Autodesk Inventor part; units mm, degrees
ref_plane "作業平面1" through (-60, -5.7151, 26) normal (0, 0, -1) x (0, 1, 0)
ref_plane "YZ Plane" through (0, 0, 0) normal (1, 0, 0) x (0, 1, 0)
ref_plane "XZ Plane" through (0, 0, 0) normal (0, 1, 0) x (-1, 0, 0)
sketch "スケッチ1" plane through (0, 0, 0) normal (0, 0, 1) x (1, 0, 0)
  circle A0 centre (-4.6538, 21.3462) radius 1.1
  circle A1 centre (-19.6538, 21.3462) radius 1.1
  line L0 (0.5, 16.7574) -> (0.5, 6.421)
  arc A2 (-3.1924, 5.3553) -> (0.5, 6.421) centre (-1.5, 6.421) ccw
  arc A3 (-3.1924, 5.3553) -> (-13.8372, 15.4455) centre (-28.2569, -10.4267) ccw
  arc A4 (-12.8636, 19.1925) -> (-13.8372, 15.4455) centre (-12.8636, 17.1925) ccw
  line L1 (-12.8636, 19.1925) -> (-2.3985, 19.1925)
  arc A5 (-1.3325, 18.8847) -> (-2.3985, 19.1925) centre (-2.3985, 17.1925) ccw
  arc A6 (-1.3325, 18.8847) -> (-0.8333, 18.643) centre (0, 21) ccw
  arc A7 (0.5, 16.7574) -> (-0.8333, 18.643) centre (-1.5, 16.7574) ccw
  arc A8 (-2.3454, -0.8655) -> (2.5, 0) centre (0, 0) ccw
  line L2 (2.5, 0) -> (2.5, 16.5)
  arc A9 (4.5, 18.5) -> (2.5, 16.5) centre (4.5, 16.5) ccw
  line L3 (4.5, 18.5) -> (21, 18.5)
  arc A10 (21, 18.5) -> (21, 23.5) centre (21, 21) ccw
  line L4 (21, 23.5) -> (-25, 23.5)
  arc A11 (-25, 23.5) -> (-59.8955, -2.5) centre (-25, -12.9173) ccw
  arc A12 (-59.8955, -2.5) -> (-55.0727, -3.8137) centre (-57.5, -3.2151) ccw
  arc A13 (-2.3454, -0.8655) -> (-55.0727, -3.8137) centre (-28.2569, -10.4267) ccw
  circle A14 centre (0, 0) radius 1.1
  circle A15 centre (-47.2894, 12.7841) radius 1.1
  circle A16 centre (-29.7988, 20.1536) radius 1.1
  circle A17 centre (0, 21) radius 1.1
  circle A18 centre (-57.5, -3.2151) radius 1.1
  circle A19 centre (21, 21) radius 1.1
  line L5 (-12.8636, 19.1925) -> (-20.8636, 19.1925)
  line L6 (-33.6212, 16.6665) -> (-20.8636, 19.1925)
  circle A20 centre (-57.5, -3.2151) radius 0.8
  circle A21 centre (-47.2894, 12.7841) radius 0.8
  circle A22 centre (-29.7988, 20.1536) radius 0.8
  circle A23 centre (-19.6538, 21.3462) radius 0.8
  circle A24 centre (-4.6538, 21.3462) radius 0.8
  circle A25 centre (-4.6538, 21.3462) radius 2.1538
  point P0 (0, 0)
  point P1 (-4.6538, 19.1925)
  point P2 (-4.6538, 23.5)
  dimension "d0" = 8
  dimension "d1" = 1.6
  dimension "d2" = 1.6
  dimension "d3" = 1.6
  dimension "d4" = 1.6
  dimension "d5" = 1.6
ref_plane "作業平面1" through (-60, -5.7151, 26) normal (0, 0, -1) x (0, 1, 0)
extrude "押し出し1" add sketch "スケッチ1" along normal up to surface (26 mm away) contours A0 | A1 | L5 L6 A13 A12 A11 L4 A25 L1 | A25 | A15 | A16 | A18
fillet "フィレット1" radius 2 1 edges at (-20.8636, 19.1925, 13)
properties part number "tesaki_sukima" material "ABS プラスチック"
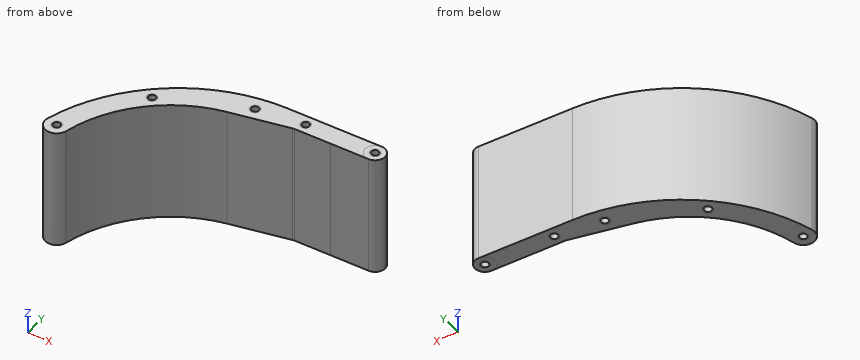
Design review of the part built by this model. Coordinates are the model's own, in mm. Coordinates: 2 decimals unless noted, no trailing zeros. Loops run counter-clockwise (first coordinate to the right, second up) from the corner with the lowest first, then second, coordinate; pieces in that order, holes last. Notation, with made-up numbers: M 56,9.25 L 94,9.25 A30 ccw 94,47.25 Z; hole C -13,-14.5 d2. An arc over 180 degrees is marked long. Answer as CSV lines item,"result".
Item 1: For probe 1 along Y at (x, z) = (-20.5, 6.25); probe 2 along X at (y, z) = (-3.5, 19); probe 3 along Y at (x, z) = (-57.5, 14.5), list the stretches that pass through material, from the lowest coordinate up.
Answer list:
probe 1,"19.19 to 23.5"
probe 2,"-59.98 to -58.25, -56.75 to -54.99"
probe 3,"-5.72 to -4.02, -2.42 to 3.51"
Item 2: Add section D-D on x = -42. State the section outline as (y, z) points.
Answer list:
outline,"M 13.53,0 L 19.29,0 L 19.29,26 L 13.53,26 Z"
Item 3: Add section B-B on z = 8.5. State the section outline as (x, y) points, plus the area to 3 significant figures.
Answer list:
outline,"M -59.9,-2.5 A2.5 ccw long -55.07,-3.81 A27.62 cw -33.62,16.67 L -21.06,19.15 A2 cw -20.67,19.19 L -4.65,19.19 A2.15 ccw -4.65,23.5 L -25,23.5 A36.42 ccw Z; hole C -57.5,-3.22 d1.6; hole C -47.29,12.78 d1.6; hole C -29.8,20.15 d1.6; hole C -19.65,21.35 d1.6; hole C -4.65,21.35 d1.6"
area,"316 mm²"
Item 4: Add section C-C on y = 0.25. State the section outline as (x, z) points, plus the area to 3 significant figures.
Answer list:
outline,"M -58.95,0 L -53.73,0 L -53.73,26 L -58.95,26 Z"
area,"136 mm²"
Item 5: For P1, Ø10, axis at x = -37, z = 22, coming from the -Y side; P2, Ø3, axis at y = 6, z = 20.5, coming from the +X side; P3, Ø2.5, axis at x = -17, z = 15, coming from the -Y side, all flat-tipped, find the tip position at first contact; note any pin that passes through.
Answer list:
P1,"y = 13.53"
P2,"x = -49.27"
P3,"y = 19.19"
Item 6: Add section A-A on x = -57.5. State the section outline as (y, z) points.
Answer list:
outline,"M -5.72,0 L -4.02,0 L -4.02,26 L -5.72,26 Z; M -2.42,0 L 3.51,0 L 3.51,26 L -2.42,26 Z"
